Verification items for the finished model (mm, model axes). Face numbers are marked on the shaded views. A direction names the side the tool comes from. Round coordinates to 2 decimals unless told otherwise and drop trailing zeros. Write each loop counter-clockwise with the first axis right and the second up, starting at its lowest first coordinate (ties: lowest second). Pieces come first, ordered by that corner, then holes. Notation, with made-up numbers: M 18.5,60.25 L 76.5,60.25 A30 ccw 76.5,99.25 Z; hole C -29,75.5 d6. An arc over 180 degrees is marked long. Answer in a Markdown table with one row per item. Add a question column.
1. Sectioned sample at C-C on x = 0. Record the cut outline in (y, z) (3 decimals), plus the area to 3 significant figures.
2. Set-up check for the marked faces 1 and 2: record each of +Z, -Z, +X, -X, +Y, -Y from which the full face is reachable in a straight line by a thin tool's end or side.
3. Draft check along Z on the marked faces 3, 4, 5 and 6. Enter one of: pulls with the +Z half, pulls with the -Z half, needs draft (parallel to the pull), parting line crosses it, or undercut.
4. Go/stop test with flat-tipped pins: pin 1 Ø1 at (x, z) = (4.5, 6.5) entering from +Y; pin 2 Ø6 at (x, z) = (-6, 17.5) entering from -Y; pin 3 Ø1.6 at (x, y) = (-0.5, 2.5) entering from +Z. Record where each tip stops, or that it passes through.
5. Sectioned sample at B-B on y = 0. Count the separate pieces of the cut face and the enclosed holes in it, plus the area to 3 significant figures.
6. Material ranges on probe 1 along X at (y, z) = (4.75, 20.5) (3 decimals); probe 2 along Z at (x, y) = (-4.25, -4) (3 decimals); probe 3 along Y at (x, z) = (-6, 22.5), recorded low to high.
7. Sectioned sample at A-A on x = -6.75. Record the cut outline in (y, z) (1 decimal), plus the area to 3 significant figures.
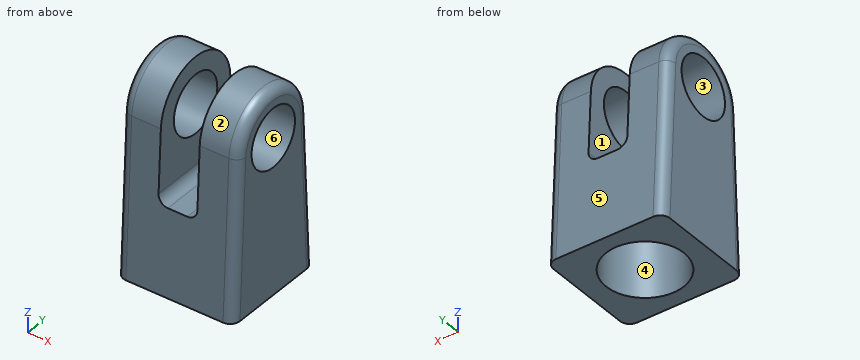
```python
from build123d import *

# Parameters (mm, degrees)
EXTRUDE2_DEPTH          = 9.525
SKETCH3_W               = 6.35
SKETCH3_H               = 19.05
CUT_EXTRUDE1_DEPTH      = 9.89
CUT_EXTRUDE1_DEPTH_BACK = 9.89
SKETCH4_R               = 4.7625
CUT_EXTRUDE2_DEPTH      = 20.05
SKETCH5_R               = 6.35
CUT_EXTRUDE3_DEPTH      = 9.525
FILLET1_R               = 1.5875


with BuildPart() as part:
    # Sketch2 → Extrude2 (new body, symmetric)
    with BuildSketch(Plane(origin=(0, 0, 0), x_dir=(0, 0, -1), z_dir=(1, 0, 0))):
        with BuildLine():
            Line((0, 8.89), (-25.777721364, 7.610632469))
            ThreePointArc((-25.777721364, 7.610632469), (-33.02, 0), (-25.777721364, -7.610632469))
            Line((-25.777721364, -7.610632469), (0, -8.89))
            Line((0, -8.89), (0, 8.89))
        make_face()
    extrude(amount=EXTRUDE2_DEPTH, both=True)

    # Sketch3 → Cut-Extrude1 (cut, two sides)
    with BuildSketch(Plane(origin=(0, 0, 0), x_dir=(1, 0, 0), z_dir=(0, 1, 0))) as cut_extrude1_sk:
        with Locations((0, -23.495)):
            Rectangle(SKETCH3_W, SKETCH3_H)
    extrude(amount=CUT_EXTRUDE1_DEPTH, mode=Mode.SUBTRACT)
    extrude(cut_extrude1_sk.sketch, amount=-CUT_EXTRUDE1_DEPTH_BACK, mode=Mode.SUBTRACT)

    # Sketch4 → Cut-Extrude2 (cut, through all)
    with BuildSketch(Plane(origin=(9.525, 0, 0), x_dir=(0, 0, -1), z_dir=(1, 0, 0))):
        with Locations((-25.4, 0)):
            Circle(SKETCH4_R)
    extrude(amount=-CUT_EXTRUDE2_DEPTH, mode=Mode.SUBTRACT)

    # Sketch5 → Cut-Extrude3 (cut)
    with BuildSketch(Plane(origin=(0, 0, 0), x_dir=(-1, 0, 0), z_dir=(0, 0, -1))):
        Circle(SKETCH5_R)
    extrude(amount=-CUT_EXTRUDE3_DEPTH, mode=Mode.SUBTRACT)

    # Fillet1
    fillet1_edges = [part.edges().sort_by_distance(p)[0] for p in [
        (9.525, 0, 33.02),
        (9.525, -8.250316234, 12.888860682),
        (-3.175, 0, 13.97),
        (3.175, 0, 13.97),
        (-9.525, -8.250316234, 12.888860682),
        (-9.525, 0, 33.02),
        (-9.525, 8.250316234, 12.888860682),
        (9.525, 8.250316234, 12.888860682),
    ]]
    fillet(fillet1_edges, radius=FILLET1_R)


solid = part.part
```
Geometry check:
| question | item | result |
|---|---|---|
| 1 | outline | M -8.89,0 L -6.35,0 L -6.35,9.525 L 6.35,9.525 L 6.35,0 L 8.89,0 L 8.197,13.97 L -8.197,13.97 Z |
| 1 | area | 118 mm2 |
| 2 | face 1 | +Z, +Y, -Y |
| 2 | face 2 | +Z, +X, -X |
| 3 | face 3 | undercut |
| 3 | face 4 | needs draft |
| 3 | face 5 | pulls with the +Z half |
| 3 | face 6 | undercut |
| 4 | pin 1 | stops at y = 8.59 |
| 4 | pin 2 | stops at y = -8.17 |
| 4 | pin 3 | stops at z = 13.97 |
| 5 | separate pieces | 3 |
| 5 | enclosed holes | 0 |
| 5 | area | 266 mm2 |
| 6 | probe 1 | x = -9.525 to -3.175, 3.175 to 9.525 |
| 6 | probe 2 | z = 9.525 to 22.815, 27.985 to 31.886 |
| 6 | probe 3 | y = -7.77 to -3.78, 3.78 to 7.77 |
| 7 | outline | M -8.9,0 L 8.9,0 L 7.6,25.8 A7.6 ccw -7.6,25.8 Z; hole C 0,25.4 d9.5 |
| 7 | area | 440 mm2 |
